Verification items for the finished model (mm, model axes). A direction names the side the tool comes from. Round coordinates to 2 decimals unless told otherwise and drop trailing zeros. One line per item, written item: value. Start each with the question number.
Autodesk Inventor part; units mm, degrees
ref_plane "Work Plane1" through (0, 6.35, 0) normal (0, 1, 0) x (-1, 0, 0)
ref_plane "YZ Plane" through (0, 0, 0) normal (1, 0, 0) x (0, 1, 0)
ref_plane "XY Plane" through (0, 0, 0) normal (0, 0, 1) x (1, 0, 0)
sketch "Sketch1" plane through (0, 0, 0) normal (0, 0, 1) x (1, 0, 0)
  line L0 (0, 0) -> (304.8, 0)
  arc A0 (304.8, 0) -> (406.4, 101.6) centre (304.8, 101.6) ccw
  line L1 (406.4, 101.6) -> (406.4, 152.4)
  line L2 (304.8, 0) -> (304.8, 101.6) construction
  line L3 (304.8, 101.6) -> (406.4, 101.6) construction
  arc A1 (406.4, 152.4) -> (304.8, 254) centre (304.8, 152.4) ccw
  line L4 (406.4, 152.4) -> (304.8, 152.4) construction
  line L5 (304.8, 152.4) -> (304.8, 254) construction
  line L6 (304.8, 254) -> (203.2, 254)
  circle A2 centre (668.9835, 281.347) radius 317.5 construction
  dimension "d0" = 304.8
  dimension "d1" = 101.6
  dimension "d2" = 50.8
  dimension "d3" = 101.6
  dimension "d4" = 101.6
  dimension "d7" = 635
sketch "Sketch2" plane through (0, 0, 0) normal (1, 0, 0) x (0, 1, 0)
  circle A0 centre (0, 0) radius 6.35
  circle A1 centre (0, 0) radius 4.7625
  dimension "d5" = 12.7
  dimension "d8" = 9.525
sweep "Sweep1" add profiles "Sketch2" path "Sketch1"
ref_plane "Work Plane1" through (0, 6.35, 0) normal (0, 1, 0) x (-1, 0, 0)
sketch "Sketch3" plane through (0, 6.35, 0) normal (0, 1, 0) x (-1, 0, 0)
  circle A0 centre (-63.5, 0) radius 2.0828
  line L0 (0, 6.35) -> (-304.8, 6.35)
  line L1 (0, -6.35) -> (-304.8, -6.35)
  line L2 (0, -6.35) -> (0, 6.35)
  circle A1 centre (-9.525, 0) radius 2.4638
  point P0 (0, 0)
  dimension "d9" = 4.1656
  dimension "d10" = 63.5
  dimension "d11" = 6.35
  dimension "d14" = 4.9276
  dimension "d15" = 9.525
  dimension "d16" = 6.35
extrude "Extrusion1" cut sketch "Sketch3" against normal blind 25.4
properties part number "Metal Pipe Clamp" material "Aluminum"
1. Scan lines: line 1 along Y through (x, z) = (25, -0.25); line 2 along X through (y, z) = (114, -0.75). Record each from-to range of solid material in increasing order.
2. Tool access check on faces 1 (the face through (400.534, 127.356, -2.432)), 2 (the face through (203.2, 249, -1)), 3 (the face through (253.289, 258.758, 0.209)). Record the directions out of +Z, -Z, +X, -X, +Y, -Y that give a thin tool (end or side, any length) a straight path to the whole face; none if there is none.
3. Depth check by flat-ended pin: pin 1 (2 mm diameter, centred on y = 22.5, z = 5, fed in from +X); pin 2 (2 mm diameter, centred on y = 164.5, z = 0.5, fed in from +X); pin 3 (4 mm diameter, centred on y = 53, z = -5, fed in from +X); pin 4 (6.5 mm diameter, centred on x = 9.525, z = 0, fed in from -Y). Enter the tip coordinate at first touch or a pass-through.
4. Draft check along Y on faces 4 (the face through (0, -5, 1)), 5 (the face through (253.289, 247.943, 1.907)), 6 (the face through (154.53, -3.78, -2.9)). Enter one of: released by +Y, released by -Y, zero draft, split by the parting line, or undercut.
5. Section check A-A (x = 232.5). Give the number of separate pieces and of enclosed holes in the cut face, and give its area (3 significant figures).
Geometry check:
1. line 1: y = -6.35 to -4.76, 4.76 to 6.35
1. line 2: x = 400.09 to 401.7, 411.1 to 412.71
2. face 1: none
2. face 2: +Z, -Z, -X, +Y
2. face 3: -X
3. pin 1: stops at x = 376.57
3. pin 2: stops at x = 412.17
3. pin 3: stops at x = 400.69
3. pin 4: stops at y = -6.35
4. face 4: zero draft
4. face 5: undercut
4. face 6: undercut
5. separate pieces: 2
5. enclosed holes: 2
5. area: 111 mm²
